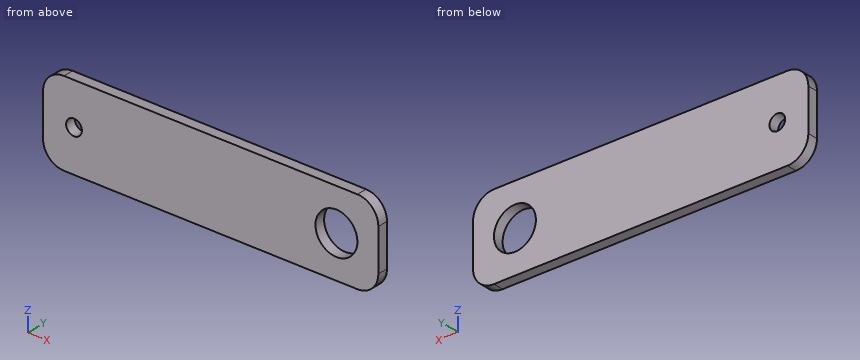
```python
from build123d import *

# Parameters (mm, degrees)
SKETCH1_W           = 50.8
SKETCH1_H           = 12.7
BOSS_EXTRUDE1_DEPTH = 1.5875
SKETCH2_R           = 1.190625
SKETCH2_R_2         = 3.175
CUT_EXTRUDE1_DEPTH  = 53.3875
FILLET1_R           = 3.175


with BuildPart() as part:
    # Sketch1 → Boss-Extrude1 (new body)
    with BuildSketch(Plane(origin=(0, 0, 0), x_dir=(1, 0, 0), z_dir=(0, 1, 0))):
        with Locations((25.4, 6.35)):
            Rectangle(SKETCH1_W, SKETCH1_H)
    extrude(amount=BOSS_EXTRUDE1_DEPTH)

    # Sketch2 → Cut-Extrude1 (cut, through all)
    with BuildSketch(Plane(origin=(0, 1.5875, 0), x_dir=(1, 0, 0), z_dir=(0, 1, 0))):
        with Locations(Location((4.699, 6.35, 0), (0, 0, 270))):
            Circle(SKETCH2_R)
        with Locations(Location((44.45, 6.35, 0), (0, 0, 270))):
            Circle(SKETCH2_R_2)
    extrude(amount=-CUT_EXTRUDE1_DEPTH, mode=Mode.SUBTRACT)

    # Fillet1
    fillet1_edges = [part.edges().sort_by_distance(p)[0] for p in [
        (0, 0.79375, -12.7),
        (50.8, 0.79375, -12.7),
        (50.8, 0.79375, 0),
        (0, 0.79375, 0),
    ]]
    fillet(fillet1_edges, radius=FILLET1_R)


solid = part.part
```
Geometry: final body of the model. Coordinates: model frame, mm. Coordinates: 2 decimals unless noted, no trailing zeros. Write each loop counter-clockwise with the first axis right and the second up, starting at its lowest first coordinate (ties: lowest second). Pieces come first, ordered by that corner, then holes. Notation, with made-up numbers: M 42,21 L 60,21 A24 cw 60,40 Z; hole C -10.75,31 d6. An arc over 180 degrees is marked long. Answer as CSV lines item,"result". Start each with the question number.
Q1. Cut plane C-C on z = -8.75. Return the cut outline in (x, y), then the cut area to 3 significant figures.
Q2. Cut plane A-A on z = -6.35. Return the cut outline in (x, y) (1 decimal).
Q3. Cut plane D-D on y = 0.6. Return the cut outline in (x, z) (3 decimals).
Q4. Line query: line 1 (X direction, y = 0.4, z = -6.35) (3 decimals); line 2 (X direction, y = 0.5, z = -6.75); line 3 (X direction, y = 0.6, z = -8.5). Output: solid intervals per line, ascending. Write a range as from..to.
Q5. Cut plane B-B on x = 44.45. Return the cut outline in (y, z) (1 decimal).
Findings below:
1,outline,"M 0,0 L 42.37,0 L 42.37,1.59 L 0,1.59 Z; M 46.53,0 L 50.8,0 L 50.8,1.59 L 46.53,1.59 Z"
1,area,"74.0 mm2"
2,outline,"M 0,0 L 3.5,0 L 3.5,1.6 L 0,1.6 Z; M 5.9,0 L 41.3,0 L 41.3,1.6 L 5.9,1.6 Z; M 47.6,0 L 50.8,0 L 50.8,1.6 L 47.6,1.6 Z"
3,outline,"M 0,-9.525 A3.175 ccw 3.175,-12.7 L 47.625,-12.7 A3.175 ccw 50.8,-9.525 L 50.8,-3.175 A3.175 ccw 47.625,0 L 3.175,0 A3.175 ccw 0,-3.175 Z; hole C 4.699,-6.35 d2.381; hole C 44.45,-6.35 d6.35"
4,line 1,"x = 0..3.508, 5.89..41.275, 47.625..50.8"
4,line 2,"x = 0..3.58, 5.82..41.3, 47.6..50.8"
4,line 3,"x = 0..42.11, 46.79..50.8"
5,outline,"M 0,-12.7 L 1.6,-12.7 L 1.6,-9.5 L 0,-9.5 Z; M 0,-3.2 L 1.6,-3.2 L 1.6,0 L 0,0 Z"
